Here's the drawing with two shaded views (mm, measured from the low corner). I have some questions. A direction names the side the tool comes from. Coordinates: 2 decimals unless noted, no trailing zeros. Write each loop counter-clockwise with the first axis right and the second up, starting at its lowest first coordinate (ties: lowest second). Pieces come first, ordered by that corner, then holes. Notation, with made-up numbers: (45, -22) -> (67, -22) arc R32 cw to (67, 14) -> close; hole circle Ø3 at (2.25, 36.25). An arc over 180 degrees is marked (long way). Put each result on its own line as item: value.
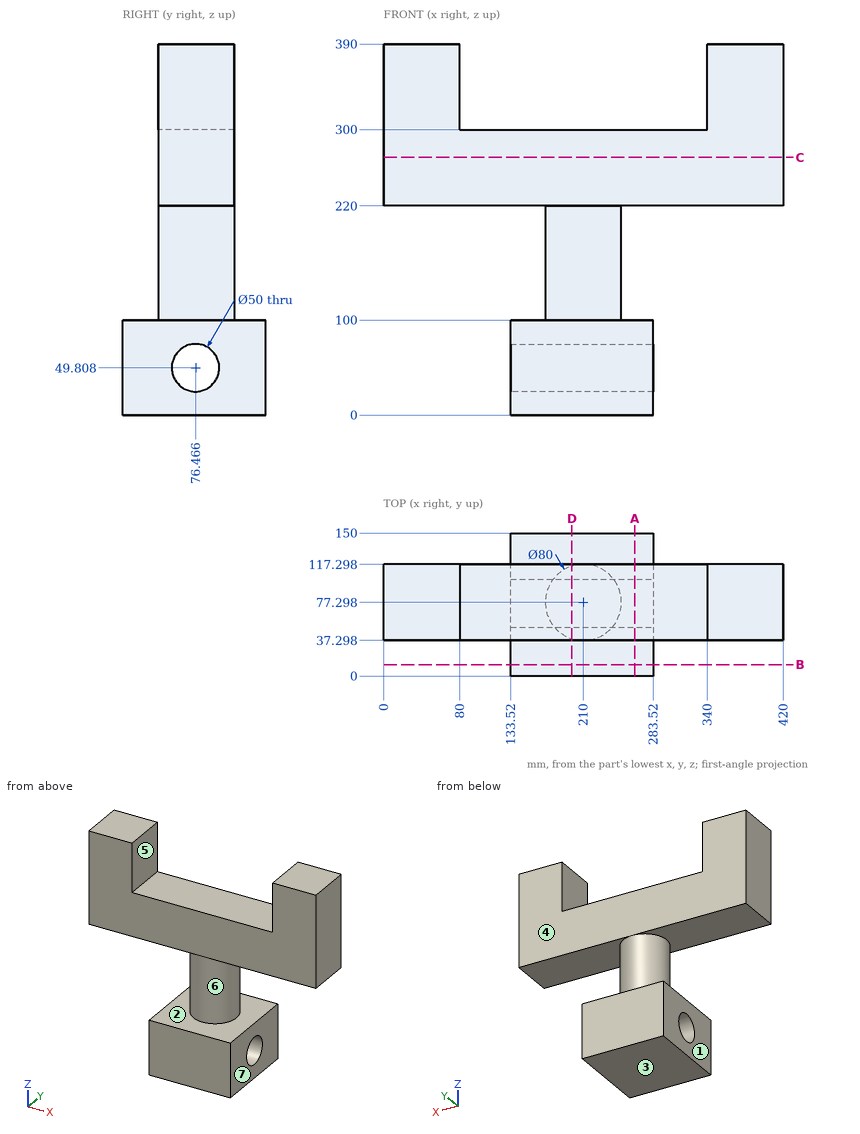
Item 1: Imagine slicing it at C-C on z = 271. Write out the boundary of the cut face in (x, y).
Output:
outline: (0, 37.3) -> (420, 37.3) -> (420, 117.3) -> (0, 117.3) -> close
Item 2: Which directions (+Z, -Z, +X, -X, +Y, -Y) give clear straight access to the entire face, cutting with the end or side of a thin tool? Please do the marked faces 4, 5, 6 and 7.
Output:
face 4: +Z, +X, -X, +Y
face 5: +Z, +Y, -Y
face 6: none
face 7: -Z, +X, +Y, -Y
Item 3: For P1, Ø5, axis at x = 227.5, z = 199.5, coming from the -Y side; P2, Ø24, axis at x = 163, y = 72.5, coming from the +Z side; P3, Ø5, axis at y = 95.5, z = 71, coming from the +X side, each with a flat end and sliding along its axis, tell me the tip position at first contact or that it passes through.
Output:
P1: stops at y = 40.22
P2: stops at z = 300
P3: stops at x = 283.52
Item 4: Please list where these lines run through material, in increasing order: line 1 along X through (y, z) = (68.5, 306); line 2 along Z through (x, y) = (274, 107.5); line 3 along Z through (x, y) = (206.5, 49). Write a range as from..to.
Output:
line 1: x = 0..80, 340..420
line 2: z = 0..100, 220..300
line 3: z = 0..300
Item 5: If we mould it in two halves opening along Z, with no side actions, what happens to the marked faces 1, 2 and 3? For each: released by +Z, released by -Z, zero draft, split by the parting line, or undercut.
Output:
face 1: zero draft
face 2: undercut
face 3: released by -Z
Item 6: Imagine slicing it at A-A on x = 264. Write out the boundary of the cut face in (y, z) (1 decimal).
Output:
outline: (0, 0) -> (150, 0) -> (150, 100) -> (0, 100) -> close; (37.3, 220) -> (117.3, 220) -> (117.3, 300) -> (37.3, 300) -> close; hole circle Ø50 at (76.5, 49.8)
Item 7: Imagine slicing it at D-D on x = 198. Write out the boundary of the cut face in (y, z) (1 decimal), then the cut area to 3 significant figures.
Output:
outline: (0, 0) -> (150, 0) -> (150, 100) -> (115.5, 100) -> (115.5, 220) -> (117.3, 220) -> (117.3, 300) -> (37.3, 300) -> (37.3, 220) -> (39.1, 220) -> (39.1, 100) -> (0, 100) -> close; hole circle Ø50 at (76.5, 49.8)
area: 28,600 mm²
Item 8: Imagine slicing it at B-B on y = 12. Write out the boundary of the cut face in (x, z).
Output:
outline: (133.52, 0) -> (283.52, 0) -> (283.52, 100) -> (133.52, 100) -> close
